The listing builds one solid part. Answer for the finished solid, in the listing's coordinates (mm). Give positions to 0.01 mm unless a question says otherwise; leave off trailing zeros. Order: outer loops, then holes, each group sorted by start corner. A loop starts at its lowest first (then second) coordinate and runs counter-clockwise, first axis right, second up. Notation, with made-up numbers: (15, 75.25) - (67, 75.25) arc R8 cw to (67, 80.25) - close; hole circle Ø1 at (47.25, -31.75). An arc over 180 degrees is marked (long way). Answer in a Markdown table with one row per item.
from build123d import *

# Parameters (mm, degrees)
F1_DEPTH   = 6.35
F4_D       = 3.7973
F4_ON_F3_D = 3.7973
F5_DEPTH   = 25.4
F6_D       = 8.001
F7_D       = 11.176


with BuildPart() as f1:
    # F0 (on Top) → F1 (new body)
    with BuildSketch(Plane.XY):
        with BuildLine():
            Line((29.8951390445, 46.4425103247), (12.1151390445, 46.4425103247))
            ThreePointArc((12.1151390445, 46.4425103247), (5.3799469537, 43.6527024155), (2.5901390445, 36.9175103247))
            ThreePointArc((2.5901390445, 36.9175103247), (5.3799469537, 30.1823182339), (12.1151390445, 27.3925103247))
            Line((12.1151390445, 27.3925103247), (29.8951390445, 27.3925103247))
            ThreePointArc((29.8951390445, 27.3925103247), (36.6303311353, 30.1823182339), (39.4201390445, 36.9175103247))
            ThreePointArc((39.4201390445, 36.9175103247), (36.6303311353, 43.6527024155), (29.8951390445, 46.4425103247))
        make_face()
        with BuildLine():
            Line((12.1151390445, 46.4425103247), (2.5901390445, 46.4425103247))
            Line((2.5901390445, 46.4425103247), (2.5901390445, 36.9175103247))
            ThreePointArc((2.5901390445, 36.9175103247), (5.3799469537, 43.6527024155), (12.1151390445, 46.4425103247))
        make_face()
        with BuildLine():
            ThreePointArc((12.1151390445, 27.3925103247), (5.3799469537, 30.1823182339), (2.5901390445, 36.9175103247))
            Line((2.5901390445, 36.9175103247), (2.5901390445, 27.3925103247))
            Line((2.5901390445, 27.3925103247), (12.1151390445, 27.3925103247))
        make_face()
        with BuildLine():
            Line((39.4201390445, 27.3925103247), (39.4201390445, 36.9175103247))
            ThreePointArc((39.4201390445, 36.9175103247), (36.6303311353, 30.1823182339), (29.8951390445, 27.3925103247))
            Line((29.8951390445, 27.3925103247), (39.4201390445, 27.3925103247))
        make_face()
        with BuildLine():
            Line((39.4201390445, 46.4425103247), (29.8951390445, 46.4425103247))
            ThreePointArc((29.8951390445, 46.4425103247), (36.6303311353, 43.6527024155), (39.4201390445, 36.9175103247))
            Line((39.4201390445, 36.9175103247), (39.4201390445, 46.4425103247))
        make_face()
    extrude(amount=-F1_DEPTH)

    # F4 (through all)
    with Locations(Plane(origin=(2.5901390445, 0, 0), x_dir=(0, -1, 0), z_dir=(-1, 0, 0))):
        with Locations((-36.9175103247, -3.175)):
            Hole(F4_D / 2)

    # F4 on F3 (through all)
    with Locations(Plane(origin=(0, 46.4425103247, 0), x_dir=(-1, 0, 0), z_dir=(0, 1, 0))):
        with Locations((-12.1151390445, -3.175), (-29.8951390445, -3.175)):
            Hole(F4_ON_F3_D / 2)

    # F0 (on Top) → F5 (cut)
    with BuildSketch(Plane.XY):
        with BuildLine():
            Line((12.1151390445, 46.4425103247), (2.5901390445, 46.4425103247))
            Line((2.5901390445, 46.4425103247), (2.5901390445, 36.9175103247))
            ThreePointArc((2.5901390445, 36.9175103247), (5.3799469537, 43.6527024155), (12.1151390445, 46.4425103247))
        make_face()
        with BuildLine():
            ThreePointArc((12.1151390445, 27.3925103247), (5.3799469537, 30.1823182339), (2.5901390445, 36.9175103247))
            Line((2.5901390445, 36.9175103247), (2.5901390445, 27.3925103247))
            Line((2.5901390445, 27.3925103247), (12.1151390445, 27.3925103247))
        make_face()
        with BuildLine():
            Line((39.4201390445, 46.4425103247), (29.8951390445, 46.4425103247))
            ThreePointArc((29.8951390445, 46.4425103247), (36.6303311353, 43.6527024155), (39.4201390445, 36.9175103247))
            Line((39.4201390445, 36.9175103247), (39.4201390445, 46.4425103247))
        make_face()
        with BuildLine():
            Line((39.4201390445, 27.3925103247), (39.4201390445, 36.9175103247))
            ThreePointArc((39.4201390445, 36.9175103247), (36.6303311353, 30.1823182339), (29.8951390445, 27.3925103247))
            Line((29.8951390445, 27.3925103247), (39.4201390445, 27.3925103247))
        make_face()
    extrude(amount=-F5_DEPTH, mode=Mode.SUBTRACT)

    # F6 (through all)
    with Locations(Plane.XY):
        with Locations((12.1151390445, 36.9564630091)):
            Hole(F6_D / 2)

    # F7 (through all)
    with Locations(Plane.XY):
        with Locations((29.8951390445, 36.9175103247)):
            Hole(F7_D / 2)


solid = f1.part
Item 1: This flat-tipped pin is pushed along its axis until it touches: P1, Ø1.5, axis at y = 43.5, z = -4.5, coming from the -X side. Where does it stop, or does it pass through?
Answer block:
| item | result |
|---|---|
| P1 | x = 4.58 |
Item 2: Find section A-A on z = -2.75. Count the separate pieces of the cut face and the enclosed holes in it, then the cut area to 3 significant figures.
Answer block:
| item | result |
|---|---|
| separate pieces | 6 |
| enclosed holes | 0 |
| area | 337 mm² |
Item 3: Consider line 1 (X direction, y = 41.5, z = -3.25); line 2 (X direction, y = 43.25, z = -3.5); line 3 (Y direction, x = 30, z = -0.5). Determine where each line is inside the solid, lowest interval first.
Answer block:
| item | result |
|---|---|
| line 1 | 3.76 to 10.22, 14.01 to 26.7, 33.09 to 38.25 |
| line 2 | 5 to 10.24, 13.99 to 28.02, 31.77 to 37.01 |
| line 3 | 27.39 to 31.33, 42.5 to 46.44 |
Item 4: Find section C-C on y = 36.5. Write down the section's boundary in (x, z).
Answer block:
| item | result |
|---|---|
| outline | (2.6, -6.35) - (8.14, -6.35) - (8.14, -5.03) - (2.6, -5.03) - close; (2.6, -1.32) - (8.14, -1.32) - (8.14, 0) - (2.6, 0) - close; (16.09, -6.35) - (24.32, -6.35) - (24.32, -5.03) - (16.09, -5.03) - close; (16.09, -1.32) - (24.32, -1.32) - (24.32, 0) - (16.09, 0) - close; (35.47, -6.35) - (39.41, -6.35) - (39.41, -5.03) - (35.47, -5.03) - close; (35.47, -1.32) - (39.41, -1.32) - (39.41, 0) - (35.47, 0) - close |
Item 5: Determine the mould class of faces 1 (the face through (21, 46.443, -3)), 2 (the face through (37.315, 38.728, -2.605)), 3 (the face through (24.73, 34.78, -3.22)), 4 (the face through (31.706, 29.497, -2.605)) for opening direction Y: pulls with the +Y half, pulls with the -Y half, needs draft (parallel to the pull), parting line crosses it, or undercut.
Answer block:
| item | result |
|---|---|
| face 1 | pulls with the +Y half |
| face 2 | undercut |
| face 3 | undercut |
| face 4 | needs draft |
